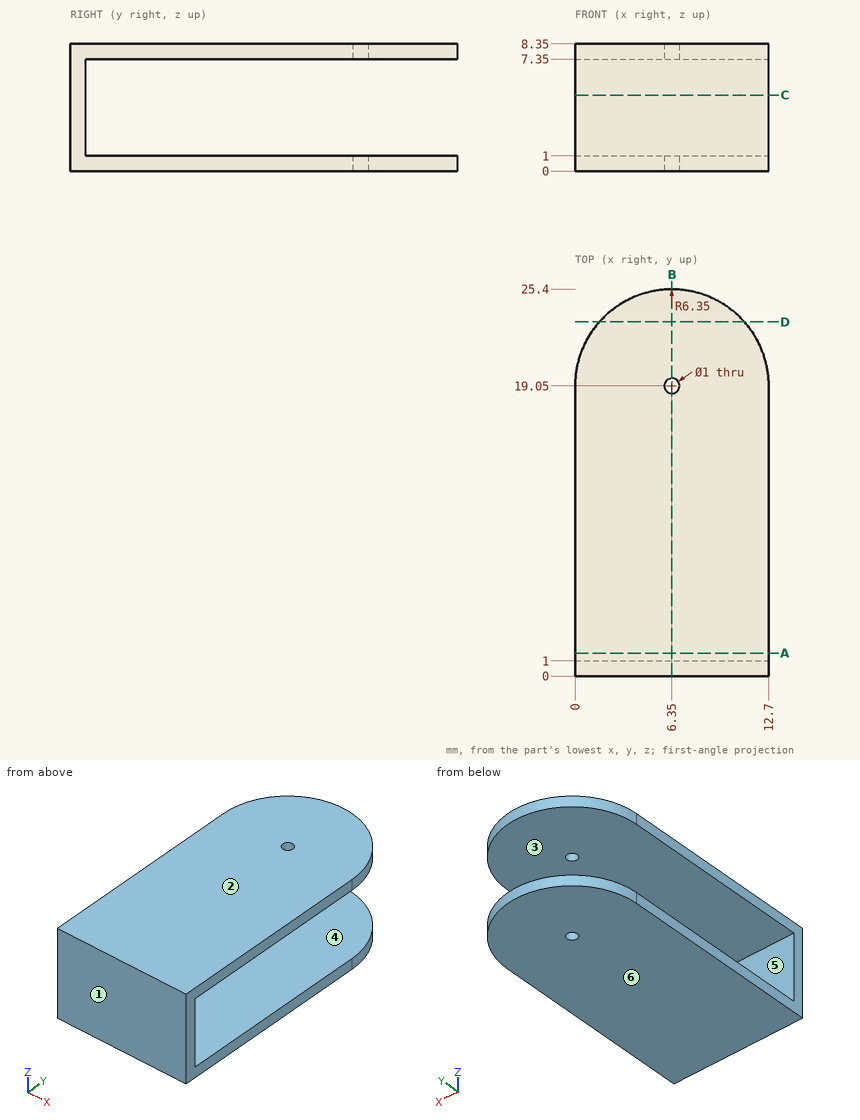
Study the drawing (mm; zero at the part's minimum x, y, z) and answer. A direction names the side the tool comes from. Coordinates: 2 decimals unless noted, no trailing zeros. Loops run counter-clockwise (first coordinate to the right, second up) from the corner with the lowest first, then second, coordinate; pieces in that order, holes last. Notation, with made-up numbers: M -5.5,75.5 L 5.5,75.5 A21 ccw 5.5,84.5 Z; hole C 84.25,-20.5 d4. An arc over 180 degrees is marked long. Answer as a JSON object with one key per item and string values. Group by question number.
Item 1: Section A-A (y = 1.5) is taken. Write down the section's boundary in (x, z).
Item 2: Section D-D (y = 23.25) is taken. Write down the section's boundary in (x, z), and give its area (3 significant figures).
Item 3: Determine the mould class of the marked faces 1, 2, 3 and 4 for opening direction Z: +Z half, -Z half, draft (parallel to the pull), parting line (faces both ways), or undercut.
Item 4: Which of the six approach directions +Z, -Z, +X, -X, +Y, -Y give full straight-line access (tool end or side, diameter ignored) to the marked faces 5 and 6?
Item 5: Section C-C (z = 5) is taken. Write down the section's boundary in (x, y), and give its area (3 significant figures).
Item 6: Consider L1, parallel to Z at x = 1.25, y = 16.25; L2, parallel to Y at x = 6.35, z = 7.7; L3, parallel to Y at x = 6.75, z = 0.5. Determine where each line is inside the solid, lowest interval first.
Item 7: Section B-B (x = 6.35) is taken. Write down the section's boundary in (y, z), and give its area (4 significant figures).
Item 8: Each of these flat-tipped pins is pushed along its axis until it touches: P1, Ø3, axis at x = 3.5, z = 4, coming from the +Y side; P2, Ø2, axis at x = 2.5, z = 1, coming from the +Y side; P3, Ø1, axis at y = 21, z = 5.5, coming from the -X side. Where does it stop, or does it pass through?
Solved:
{
 "1": {"outline": "M 0,0 L 12.7,0 L 12.7,1 L 0,1 Z; M 0,7.35 L 12.7,7.35 L 12.7,8.35 L 0,8.35 Z"},
 "2": {"outline": "M 1.59,0 L 11.11,0 L 11.11,1 L 1.59,1 Z; M 1.59,7.35 L 11.11,7.35 L 11.11,8.35 L 1.59,8.35 Z", "area": "19.1 mm2"},
 "3": {"face 1": "draft", "face 2": "+Z half", "face 3": "undercut", "face 4": "undercut"},
 "4": {"face 5": "+X, -X, +Y", "face 6": "-Z, +X, -X, +Y, -Y"},
 "5": {"outline": "M 0,0 L 12.7,0 L 12.7,1 L 0,1 Z", "area": "12.7 mm2"},
 "6": {"L1": "z = 0 to 1, 7.35 to 8.35", "L2": "y = 0 to 18.55, 19.55 to 25.4", "L3": "y = 0 to 18.75, 19.35 to 25.39"},
 "7": {"outline": "M 0,0 L 18.55,0 L 18.55,1 L 1,1 L 1,7.35 L 18.55,7.35 L 18.55,8.35 L 0,8.35 Z; M 19.55,0 L 25.4,0 L 25.4,1 L 19.55,1 Z; M 19.55,7.35 L 25.4,7.35 L 25.4,8.35 L 19.55,8.35 Z", "area": "55.15 mm2"},
 "8": {"P1": "stops at y = 1", "P2": "stops at y = 24.72", "P3": "passes through"}
}
